Could you check a few things on this model? Use its own coordinates, in mm. Give positions to 0.01 mm unless a question says otherwise; leave off trailing zeros. Write each loop counter-clockwise with the first axis right and the second up, starting at its lowest first coordinate (ties: lowest second). Pieces come first, ordered by that corner, then holes. Notation, with made-up numbers: (34.5, 26.5) - (73.5, 26.5) arc R18 cw to (73.5, 61.5) - close; hole circle Ø10 at (-31.75, 37.25). An arc over 180 degrees is marked (long way). Write item = value, one per line.
from build123d import *

# Parameters (mm, degrees)
F0_W     = 85.09
F0_H     = 85.09
F0_R     = 2.5
F1_DEPTH = 7.62
F2_W     = 80.01
F2_H     = 80.01
F3_DEPTH = 5.08


with BuildPart() as f1:
    # F0 (on Front) → F1 (new body)
    with BuildSketch(Plane.XZ):
        with Locations((40.005, 40.005)):
            Rectangle(F0_W, F0_H)
        with Locations((4, 4)):
            Circle(F0_R, mode=Mode.SUBTRACT)
        with Locations((76.01, 4)):
            Circle(F0_R, mode=Mode.SUBTRACT)
        with BuildLine():
            ThreePointArc((25.4, 0), (7.439488, 7.439488), (0, 25.4))
            Line((0, 25.4), (0, 80.01))
            Line((0, 80.01), (80.01, 80.01))
            Line((80.01, 80.01), (80.01, 25.4))
            ThreePointArc((80.01, 25.4), (72.570512, 7.439488), (54.61, 0))
            Line((54.61, 0), (25.4, 0))
        make_face(mode=Mode.SUBTRACT)
    extrude(amount=F1_DEPTH)

    # F2 (on face) → F3 (cut)
    with BuildSketch(Plane(origin=(0, 0, 0), x_dir=(-1, 0, 0), z_dir=(0, 1, 0))):
        with Locations((-40.005, 40.005)):
            Rectangle(F2_W, F2_H)
    extrude(amount=-F3_DEPTH, mode=Mode.SUBTRACT)


solid = f1.part
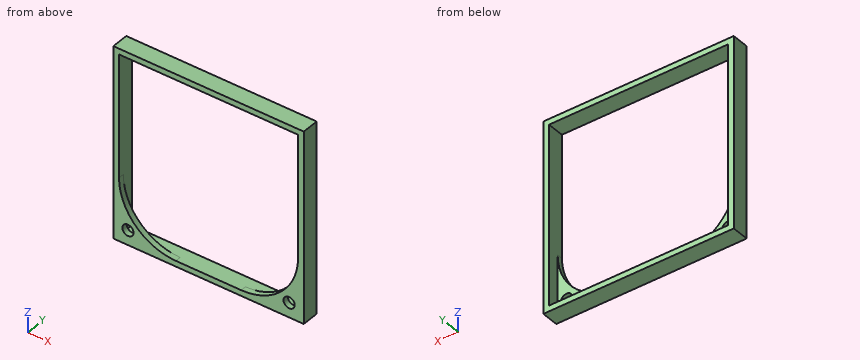
1. I need wall thicknesses on line 1 (Z direction, x = 55, y = -3.5); line 2 (X direction, y = -6.9, z = 4). Which ranges of each line are inside material? Lowest first, please.
Filled sheet:
line_1 = -2.54 to 0, 80.01 to 82.55
line_2 = -2.54 to 1.5, 6.5 to 11.72, 68.29 to 73.51, 78.51 to 82.55
2. For pin 1 (7.5 mm diameter, centred on x = 71, z = 14.5, fed in from +Y), with a flat end and sliding along its axis, tell me the tip position at first contact or that it passes through.
Filled sheet:
pin_1 = through
3. If we section it at B-B, the plane x = 29.5: Please give me the cut outline in (y, z).
Filled sheet:
outline = (-7.62, -2.54) - (0, -2.54) - (0, 0) - (-7.62, 0) - close; (-7.62, 80.01) - (0, 80.01) - (0, 82.55) - (-7.62, 82.55) - close
4. If we section it at A-A, the plane z = 71: Please give me the cut outline in (x, y), and give its area (3 significant figures).
Filled sheet:
outline = (-2.54, -7.62) - (0, -7.62) - (0, 0) - (-2.54, 0) - close; (80.01, -7.62) - (82.55, -7.62) - (82.55, 0) - (80.01, 0) - close
area = 38.7 mm2
5. If we section it at D-D, the plane z = 4: Please give me the cut outline in (x, y), and give its area (3 significant figures).
Filled sheet:
outline = (-2.54, -7.62) - (1.5, -7.62) - (1.5, -5.08) - (0, -5.08) - (0, 0) - (-2.54, 0) - close; (6.5, -7.62) - (11.72, -7.62) - (11.72, -5.08) - (6.5, -5.08) - close; (68.29, -7.62) - (73.51, -7.62) - (73.51, -5.08) - (68.29, -5.08) - close; (78.51, -7.62) - (82.55, -7.62) - (82.55, 0) - (80.01, 0) - (80.01, -5.08) - (78.51, -5.08) - close
area = 72.8 mm2
6. If we section it at C-C, the plane y = -3.75: Please give me the cut outline in (x, z).
Filled sheet:
outline = (-2.54, -2.54) - (82.55, -2.54) - (82.55, 82.55) - (-2.54, 82.55) - close; hole (0, 0) - (80.01, 0) - (80.01, 80.01) - (0, 80.01) - close
